The model under review builds one solid part; all positions refer to its coordinate system, in mm. A direction names the side the tool comes from. Coordinates: 2 decimals unless noted, no trailing zeros. Order: outer loops, then holes, each group sorted by start corner. A loop starts at its lowest first (then second) coordinate and runs counter-clockwise, first axis right, second up. Notation, with made-up numbers: (0, 61) -> (30, 61) arc R25 ccw to (30, 81) -> close; hole circle Ø2 at (25, -24.75). An arc over 180 degrees is marked (long way). Put each result on its own line as item: value.
from build123d import *

# Parameters (mm, degrees)
SKETCH_1_R      = 2.5
EXTRUDE_1_DEPTH = 3
SKETCH_2_R      = 2.5
EXTRUDE_2_DEPTH = 2
SKETCH_3_W      = 1.5
SKETCH_3_H      = 20
EXTRUDE_4_DEPTH = 3
SKETCH_5_W      = 1.5
SKETCH_5_H      = 20
REVOLVE_2_ANGLE = 90
SKETCH_6_W      = 1.5
SKETCH_6_H      = 20
EXTRUDE_5_DEPTH = 5
SKETCH_8_W      = 1.5
SKETCH_8_H      = 20
REVOLVE_3_ANGLE = 90
SKETCH_9_W      = 1.5
SKETCH_9_H      = 20
EXTRUDE_6_DEPTH = 5


with BuildPart() as part:
    # 草图1 → 凸台-拉伸1 (new body)
    with BuildSketch(Plane.XY):
        with BuildLine():
            Line((-25, 30), (25, 30))
            ThreePointArc((25, 30), (28.535533906, 28.535533906), (30, 25))
            Line((30, 25), (30, -25))
            ThreePointArc((30, -25), (28.535533906, -28.535533906), (25, -30))
            Line((25, -30), (-25, -30))
            ThreePointArc((-25, -30), (-28.535533906, -28.535533906), (-30, -25))
            Line((-30, -25), (-30, 25))
            ThreePointArc((-30, 25), (-28.535533906, 28.535533906), (-25, 30))
        make_face()
        with Locations((-25, 25)):
            Circle(SKETCH_1_R, mode=Mode.SUBTRACT)
        with Locations(Location((25, 25, 0), (0, 0, 180))):
            Circle(SKETCH_1_R, mode=Mode.SUBTRACT)
        with Locations((25, -25)):
            Circle(SKETCH_1_R, mode=Mode.SUBTRACT)
        with Locations(Location((-25, -25, 0), (0, 0, 180))):
            Circle(SKETCH_1_R, mode=Mode.SUBTRACT)
    extrude(amount=EXTRUDE_1_DEPTH)

    # 草图2 → 凸台-拉伸2 (add)
    # profile 1 of 4: a face of its own
    with BuildSketch(Plane.XY.offset(3)):
        with BuildLine():
            Line((-30, 25), (-30, 20))
            Line((-30, 20), (-20, 20))
            Line((-20, 20), (-20, 30))
            Line((-20, 30), (-25, 30))
            ThreePointArc((-25, 30), (-28.535533906, 28.535533906), (-30, 25))
        make_face()
        with Locations((-25, 25)):
            Circle(SKETCH_2_R, mode=Mode.SUBTRACT)
    # profile 2 of 4: a face of its own
    with BuildSketch(Plane.XY.offset(3)):
        with BuildLine():
            Line((20, 30), (25, 30))
            ThreePointArc((25, 30), (28.535533906, 28.535533906), (30, 25))
            Line((30, 25), (30, 20))
            Line((30, 20), (20, 20))
            Line((20, 20), (20, 30))
        make_face()
        with Locations(Location((25, 25, 0), (0, 0, 180))):
            Circle(SKETCH_2_R, mode=Mode.SUBTRACT)
    # profile 3 of 4: a face of its own
    with BuildSketch(Plane.XY.offset(3)):
        with BuildLine():
            Line((30, -25), (30, -20))
            Line((30, -20), (20, -20))
            Line((20, -20), (20, -30))
            Line((20, -30), (25, -30))
            ThreePointArc((25, -30), (28.535533906, -28.535533906), (30, -25))
        make_face()
        with Locations((25, -25)):
            Circle(SKETCH_2_R, mode=Mode.SUBTRACT)
    # profile 4 of 4: a face of its own
    with BuildSketch(Plane.XY.offset(3)):
        with BuildLine():
            Line((-20, -30), (-25, -30))
            ThreePointArc((-25, -30), (-28.535533906, -28.535533906), (-30, -25))
            Line((-30, -25), (-30, -20))
            Line((-30, -20), (-20, -20))
            Line((-20, -20), (-20, -30))
        make_face()
        with Locations(Location((-25, -25, 0), (0, 0, 180))):
            Circle(SKETCH_2_R, mode=Mode.SUBTRACT)
    extrude(amount=EXTRUDE_2_DEPTH)

    # 草图3 → 凸台-拉伸4 (add)
    with BuildSketch(Plane(origin=(0, 0, 0), x_dir=(-1, 0, 0), z_dir=(0, 0, -1))):
        with Locations((-12.75, 0)):
            Rectangle(SKETCH_3_W, SKETCH_3_H)
        with Locations((12.75, 0)):
            Rectangle(SKETCH_3_W, SKETCH_3_H)
    extrude(amount=EXTRUDE_4_DEPTH)

    # 草图5 → 旋转2 (revolve)
    with BuildSketch(Plane(origin=(0, 0, -3), x_dir=(-1, 0, 0), z_dir=(0, 0, -1))):
        with Locations((-12.75, 0)):
            Rectangle(SKETCH_5_W, SKETCH_5_H)
    revolve(axis=Axis((12, 10, -3), (0, 1, 0)), revolution_arc=REVOLVE_2_ANGLE)

    # 草图6 → 凸台-拉伸5 (add)
    with BuildSketch(Plane.ZY.offset(-12)):
        with Locations((-3.75, 0)):
            Rectangle(SKETCH_6_W, SKETCH_6_H)
    extrude(amount=EXTRUDE_5_DEPTH)

    # 草图8 → 旋转3 (revolve)
    with BuildSketch(Plane(origin=(0, 0, -3), x_dir=(-1, 0, 0), z_dir=(0, 0, -1))):
        with Locations((12.75, 0)):
            Rectangle(SKETCH_8_W, SKETCH_8_H)
    revolve(axis=Axis((-12, 10, -3), (0, -1, 0)), revolution_arc=REVOLVE_3_ANGLE)

    # 草图9 → 凸台-拉伸6 (add)
    with BuildSketch(Plane(origin=(-12, 0, 0), x_dir=(0, 0, -1), z_dir=(1, 0, 0))):
        with Locations((3.75, 0)):
            Rectangle(SKETCH_9_W, SKETCH_9_H)
    extrude(amount=EXTRUDE_6_DEPTH)


solid = part.part
Item 1: Consider section B-B on x = -9. Write out the cut boundary in (y, z).
Answers below:
outline: (-30, 0) -> (30, 0) -> (30, 3) -> (-30, 3) -> close; (-10, -4.5) -> (10, -4.5) -> (10, -3) -> (-10, -3) -> close
Item 2: For pin 1 Ø1.3 at (x, z) = (10, -1.5) entering from -Y; pin 2 Ø4 at (x, y) = (17, -22) entering from -Z; pin 3 Ø8 at (x, y) = (-25, -25) entering from +Z; pin 4 Ø0.6 at (y, z) = (-26.5, 4) entering from +X, all flat-tipped, find the tip position at first contact; note any pin that passes through.
Answers below:
pin 1: through
pin 2: z = 0
pin 3: z = 5
pin 4: x = 29.85
Item 3: For line 1 (Y direction, x = 25, z = 3.45); line 2 (Y direction, x = 25, z = 2.25); line 3 (X direction, y = -7, z = -2), list the stretches that pass through material, from the lowest coordinate up. Write a range as from..to.
Answers below:
line 1: -30..-27.5, -22.5..-20, 20..22.5, 27.5..30
line 2: -30..-27.5, -22.5..22.5, 27.5..30
line 3: -13.5..-12, 12..13.5
Item 4: For faces 1 (the flat face through (-10, 0, -3)), 2 (the flat face through (-11, -10, -3.2)), 3 (the flat face through (25, 20, 4)), list the 3-axis set-ups (+Z, -Z, +X, -X, +Y, -Y) from which the entire face can be reached by the end or side of a thin tool; tool diameter is ignored.
Answers below:
face 1: +Y, -Y
face 2: -Z, +X, -X, -Y
face 3: +Z, +X, -X
Item 5: Consider section A-A on z = -1.5. Write out the cut boundary in (x, y).
Answers below:
outline: (-13.5, -10) -> (-12, -10) -> (-12, 10) -> (-13.5, 10) -> close; (12, -10) -> (13.5, -10) -> (13.5, 10) -> (12, 10) -> close
Item 6: Consider section D-D on x = 5. Write out the cut boundary in (y, z).
Answers below:
outline: (-30, 0) -> (30, 0) -> (30, 3) -> (-30, 3) -> close
Item 7: Consider section C-C on y = -21. Write out the cut boundary in (x, z).
Answers below:
outline: (-30, 0) -> (30, 0) -> (30, 5) -> (20, 5) -> (20, 3) -> (-20, 3) -> (-20, 5) -> (-30, 5) -> close
Item 8: Mouldability with a two-part tool opening along X and no side actions: class faces 4 (the flat face through (0, -30, 2)), 5 (the flat face through (30, 0, 2)), 6 (the flat face through (-20, -25, 4)) as +X half, -X half, draft (parallel to the pull), parting line (faces both ways), or undercut.
Answers below:
face 4: draft
face 5: +X half
face 6: undercut
